Read the model definition and answer for the solid it produces. Units are mm, in the model's axes. Face numbers are marked on the shaded views. Give positions to 0.01 mm unless a question says otherwise; leave off trailing zeros. Write each loop counter-clockwise with the first axis right and the second up, starting at its lowest first coordinate (ties: lowest second). Pieces come first, ordered by that corner, then holes. Notation, with made-up numbers: (-15.5, -16) - (10.5, -16) arc R36 ccw to (10.5, 20) - close; hole circle Ø6 at (13, 55.25). An arc over 180 degrees is marked (long way). Answer as a JSON object with one key per item and string values. Group by question number.
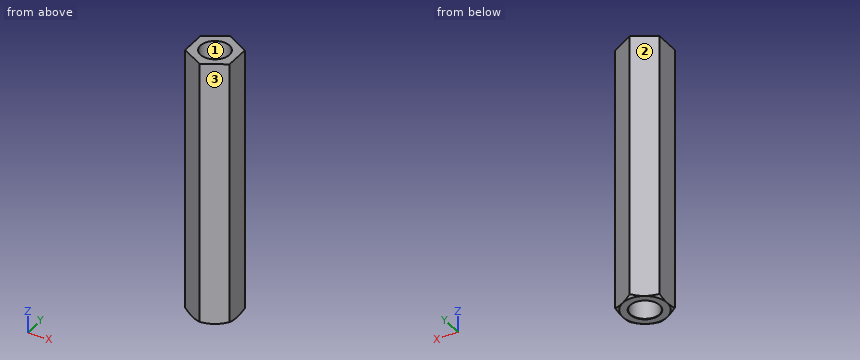
```python
from build123d import *

# Parameters (mm, degrees)
EXTRUDE1_DEPTH      = 19.05
EXTRUDE1_DEPTH_BACK = 19.05
SKETCH1_R           = 2.0828
SKETCH8_OUTSIDE_W   = 152.724
SKETCH8_OUTSIDE_H   = 153.706
SKETCH8_OUTSIDE_R   = 3.175
EXTRUDE4_DEPTH      = 39.407440143
EXTRUDE4_DRAFT      = -60


with BuildPart() as part:
    # Sketch1 → Extrude1 (new, two sides: drawn at the far end of the back side and taken through both)
    with BuildSketch(Plane.XY.offset(-EXTRUDE1_DEPTH_BACK)):
        Polygon((0, 3.666174209), (-3.175, 1.833087105), (-3.175, -1.833087105), (0, -3.666174209), (3.175, -1.833087105), (3.175, 1.833087105), align=None)
        with Locations(Location((0, 0, 0), (0, 0, 180))):
            Circle(SKETCH1_R, mode=Mode.SUBTRACT)
    extrude(amount=EXTRUDE1_DEPTH + EXTRUDE1_DEPTH_BACK)

    # Extrude3 cone 1 section (through the dimple's axis) → Extrude3 (revolve, cut)
    with BuildSketch(Plane(origin=(0, 0, -19.05), x_dir=(0, 1, 0), z_dir=(1, 0, 0))):
        Polygon((0, 0), (2.1336, 0), (0, 2.28800588), align=None)
    revolve(axis=Axis((0, 0, -19.05), (0, 0, 1)), mode=Mode.SUBTRACT)


with BuildPart() as extrude4_tool:
    # Sketch8 outside → Extrude4 (with draft: the straight prism first)
    with BuildSketch(Plane(origin=(0, 0, -19.05), x_dir=(-1, 0, 0), z_dir=(0, 0, -1))):
        Rectangle(SKETCH8_OUTSIDE_W, SKETCH8_OUTSIDE_H)
        Circle(SKETCH8_OUTSIDE_R, mode=Mode.SUBTRACT)
    extrude(amount=-EXTRUDE4_DEPTH)
    # Extrude4: the draft: its side faces are tilted about the plane it starts from
    extrude4_sides = [extrude4_tool.faces().sort_by_distance(p)[0] for p in [
        (0, -76.853, 0.653720071),
        (-76.362, 0, 0.653720071),
        (0, 76.853, 0.653720071),
        (76.362, 0, 0.653720071),
        (3.175, 0, 0.653720071),
    ]]
    draft(extrude4_sides, Plane(origin=(0, 0, -19.05), x_dir=(-1, 0, 0), z_dir=(0, 0, -1)), EXTRUDE4_DRAFT)


with BuildPart() as part_1:
    add(part.part)

    # Extrude4: cut by extrude4_tool
    add(extrude4_tool.part, mode=Mode.SUBTRACT)


solid = part_1.part
```
1) A flat-ended cylindrical pin translates along its axis: pin 1 Ø1 at (y, z) = (2.5, -11.5) entering from -X. Find the tip coordinate at first contact, or state that the pin passes through.
2) Find the intervals of material crossed by line 1 (X direction, y = 1, z = -14.5) (3 decimals); line 2 (Y direction, x = -1.5, z = -16); line 3 (Y direction, x = -1, z = -12), in increasing order. Write a range as [from, to].
3) For a pull along X with two mould halves and no side action, classify the marked faces 1, 2 and 3 as released by +X, released by -X, zero draft, split by the parting line, or undercut.
4) Find section A-A, the plane z = 13. Write down the section's boundary in (x, y) (3 decimals), and give its area (3 significant figures).
Values follow:
{
 "1": {"pin 1": "stops at x = -2.89"},
 "2": {"line 1": "x = [-3.175, -1.827], [1.827, 3.175]", "line 2": "y = [-2.8, -1.45], [1.45, 2.8]", "line 3": "y = [-3.09, -1.83], [1.83, 3.09]"},
 "3": {"face 1": "undercut", "face 2": "released by -X", "face 3": "released by +X"},
 "4": {"outline": "(-3.175, -1.833) - (0, -3.666) - (3.175, -1.833) - (3.175, 1.833) - (0, 3.666) - (-3.175, 1.833) - close; hole circle Ø4.166 at (0, 0)", "area": "21.3 mm2"}
}
